Autodesk Inventor part; units mm, degrees
ref_plane "din_908_XY" through (0, 0, 0) normal (0, 1, 0) x (1, 0, 0)
ref_plane "din_908_YZ" through (0, 0, 0) normal (1, 0, 0) x (0, 0, -1)
ref_plane "din_908_ZX" through (0, 0, 0) normal (0, 0, -1) x (0, 1, 0)
sketch "Sketch_1" plane through (0, 0, 0) normal (0, 0, 1) x (1, 0, 0)
  line L0 (0, -5.3) -> (0, 2.5)
  line L1 (0, 2.5) -> (4.45, 2.5)
  line L2 (4.45, 2.5) -> (4.75, 2.2)
  line L3 (4.75, 2.2) -> (4.75, 0.3)
  line L4 (4.75, 0.3) -> (4.45, 0)
  line L5 (4.45, 0) -> (3.5, 0)
  line L6 (3.5, 0) -> (3.5, -4.8)
  line L7 (3.5, -4.8) -> (3, -5.3)
  line L8 (3, -5.3) -> (0, -5.3)
  line L9 (0, -5.3) -> (0, 2.5)
revolve "Revolution1" add sketch "Sketch_1" angle 360 about axis through (0, -5.3, 0) along (0, -1, 0)
thread "Thread1"
sketch "Sketch_4" plane through (0, 2.5, 0) normal (0, 1, 0) x (1, 0, 0)
  line L0 (-1.5, -0.866) -> (0, -1.7321)
  line L1 (0, -1.7321) -> (1.5, -0.866)
  line L2 (1.5, -0.866) -> (1.5, 0.866)
  line L3 (1.5, 0.866) -> (0, 1.7321)
  line L4 (0, 1.7321) -> (-1.5, 0.866)
  line L5 (-1.5, 0.866) -> (-1.5, -0.866)
extrude "Extrusion1" cut sketch "Sketch_4" against normal blind 2.5
ref_plane "din_908_XY" through (0, 0, 0) normal (0, 1, 0) x (1, 0, 0)
ref_plane "din_908_YZ" through (0, 0, 0) normal (1, 0, 0) x (0, 0, -1)
ref_plane "din_908_ZX" through (0, 0, 0) normal (0, 0, -1) x (0, 1, 0)
properties part number "Verschlussschraube DIN908 M7"
The listing builds one solid part. Answer for the finished solid, in the listing's coordinates (mm). A direction names the side the tool comes from. Give positions to 0.01 mm unless a question says otherwise; leave off trailing zeros. Write each loop counter-clockwise with the first axis right and the second up, starting at its lowest first coordinate (ties: lowest second). Pieces come first, ordered by that corner, then holes.
1) For a pull along Z with two mould halves and no side action, classify faces 4 (the face through (0.74, 1.268, 1.305)), 5 (the face through (2.192, 1.237, -4.214)), 6 (the face through (2, 2.5, 0)), 7 (the face through (0.76, 1.268, -1.293)) as pulls with the +Z half, pulls with the -Z half, needs draft (parallel to the pull), parting line crosses it, or undercut.
2) Section B-B (z = 0) is taken. Write down the section's boundary in (x, y), and give its area (3 significant figures).
3) Section C-C (y = -3) is taken. Write down the section's boundary in (x, z), and give its area (3 significant figures).
4) Given P1, Ø4, axis at y = -2.5, z = 0.5, coming from the -X side; P2, Ø0.9, axis at x = 0.5, z = 0, coming from the +Y side, each flat-ended and moving along its own axis, determine where each tip first touches the part or whether it passes through.
5) A tool of negligible diameter and unlimited length cuts with its end or side. For faces 1 (the face through (0, -5.3, 0)), 2 (the face through (-0.76, 1.268, 1.293)), 3 (the face through (3.233, -2.434, -1.341)), from which of +Z, -Z, +X, -X, +Y, -Y can it reach the whole face along a straight path? Write none if from no direction.
6) Find the intervals of material crossed by L1, parallel to Y at x = 3.5, z = 2.5; L2, parallel to Y at x = -0.75, z = -0.25; L3, parallel to X at y = 1.75, z = -1, in increasing order.
7) Section A-A (y = 1.25) is taken. Write down the section's boundary in (x, z).
Response:
1. face 4: undercut
1. face 5: parting line crosses it
1. face 6: needs draft
1. face 7: undercut
2. outline: (-4.75, 0.3) - (-4.45, 0) - (-3.5, 0) - (-3.5, -4.8) - (-3, -5.3) - (3, -5.3) - (3.5, -4.8) - (3.5, 0) - (4.45, 0) - (4.75, 0.3) - (4.75, 2.2) - (4.45, 2.5) - (1.5, 2.5) - (1.5, 0) - (-1.5, 0) - (-1.5, 2.5) - (-4.45, 2.5) - (-4.75, 2.2) - close
2. area: 52.9 mm2
3. outline: circle Ø7 at (0, 0)
3. area: 38.5 mm2
4. P1: stops at x = -3.5
4. P2: stops at y = 0
5. face 1: +Z, -Z, +X, -X, -Y
5. face 2: +Y
5. face 3: -Y
6. L1: y = 0 to 2.5
6. L2: y = -5.3 to 0
6. L3: x = -4.64 to -1.27, 1.27 to 4.64
7. outline: circle Ø9.5 at (0, 0); hole (-1.5, -0.87) - (0, -1.73) - (1.5, -0.87) - (1.5, 0.87) - (0, 1.73) - (-1.5, 0.87) - close
